from build123d import *

# Parameters (mm, degrees)
SKETCH_1_R          = 7.5
EXTRUDE_1_DEPTH     = 1
FILLET_1_R          = 3
FILLET_2_R          = 3.5
CUT_EXTRUDE_1_DEPTH = 10
EXTRUDE_2_DEPTH     = 1
FILLET_3_R          = 5


with BuildPart() as part:
    # 草图1 → 凸台-拉伸1 (new body)
    with BuildSketch(Plane.XY):
        with BuildLine():
            Line((-34, 37.637190605), (-34, 37.66227766))
            ThreePointArc((-34, 37.66227766), (-35.458039892, 36.370828693), (-36, 34.5))
            Line((-36, 34.5), (-36, -12))
            Line((-36, -12), (-41, -17))
            Line((-41, -17), (-41, -37))
            Line((-41, -37), (-36, -42))
            Line((-36, -42), (-36, -48.5))
            ThreePointArc((-36, -48.5), (-34.974873734, -50.974873734), (-32.5, -52))
            Line((-32.5, -52), (-3, -52))
            Line((-3, -52), (27, -52))
            Line((27, -52), (27, -30.660254038))
            Line((27, -30.660254038), (22, -22))
            Line((22, -22), (22, -2))
            Line((22, -2), (22, 37.977350269))
            Line((22, 37.977350269), (-32.5, 37.977350269))
            ThreePointArc((-32.5, 37.977350269), (-33.269043009, 37.891244277), (-34, 37.637190605))
        make_face()
        Circle(SKETCH_1_R, mode=Mode.SUBTRACT)
        with BuildLine():
            Line((-38, -34.5), (-37, -34.5))
            ThreePointArc((-37, -34.5), (-36.292893219, -34.207106781), (-36, -33.5))
            Line((-36, -33.5), (-36, -20.5))
            ThreePointArc((-36, -20.5), (-36.292893219, -19.792893219), (-37, -19.5))
            Line((-37, -19.5), (-38, -19.5))
            ThreePointArc((-38, -19.5), (-38.707106781, -19.792893219), (-39, -20.5))
            Line((-39, -20.5), (-39, -33.5))
            ThreePointArc((-39, -33.5), (-38.707106781, -34.207106781), (-38, -34.5))
        make_face(mode=Mode.SUBTRACT)
        with BuildLine():
            Line((-14.5, -46.5), (-9.5, -46.5))
            ThreePointArc((-9.5, -46.5), (1.813708499, -41.813708499), (6.5, -30.5))
            Line((6.5, -30.5), (6.5, -24.5))
            ThreePointArc((6.5, -24.5), (1.813708499, -13.186291501), (-9.5, -8.5))
            Line((-9.5, -8.5), (-14.5, -8.5))
            ThreePointArc((-14.5, -8.5), (-25.813708499, -13.186291501), (-30.5, -24.5))
            Line((-30.5, -24.5), (-30.5, -30.5))
            ThreePointArc((-30.5, -30.5), (-25.813708499, -41.813708499), (-14.5, -46.5))
        make_face(mode=Mode.SUBTRACT)
        with BuildLine():
            Line((11.977350269, 31), (11.977350269, 18.384776311))
            ThreePointArc((11.977350269, 18.384776311), (11.370110637, 15.331976529), (9.640838471, 12.74393784))
            Line((9.640838471, 12.74393784), (7.791596066, 10.894695435))
            ThreePointArc((7.791596066, 10.894695435), (7.199175676, 9.464466094), (7.791596066, 8.034236753))
            Line((7.791596066, 8.034236753), (8.498702848, 7.327129972))
            ThreePointArc((8.498702848, 7.327129972), (9.928932188, 6.734709582), (11.359161529, 7.327129972))
            Line((11.359161529, 7.327129972), (14.672870028, 10.640838471))
            ThreePointArc((14.672870028, 10.640838471), (16.411961883, 13.243573363), (17.022649731, 16.313708499))
            Line((17.022649731, 16.313708499), (17.022649731, 31))
            ThreePointArc((17.022649731, 31), (16.430229341, 32.430229341), (15, 33.022649731))
            Line((15, 33.022649731), (14, 33.022649731))
            ThreePointArc((14, 33.022649731), (12.569770659, 32.430229341), (11.977350269, 31))
        make_face(mode=Mode.SUBTRACT)
        with BuildLine():
            Line((7, 33.022649731), (2, 33.022649731))
            ThreePointArc((2, 33.022649731), (0.569770659, 32.430229341), (-0.022649731, 31))
            Line((-0.022649731, 31), (-0.022649731, 12.328427125))
            ThreePointArc((-0.022649731, 12.328427125), (1.225965459, 10.459742437), (3.430229341, 10.898197784))
            Line((3.430229341, 10.898197784), (6.672870028, 14.140838471))
            ThreePointArc((6.672870028, 14.140838471), (8.411961883, 16.743573363), (9.022649731, 19.813708499))
            Line((9.022649731, 19.813708499), (9.022649731, 31))
            ThreePointArc((9.022649731, 31), (8.430229341, 32.430229341), (7, 33.022649731))
        make_face(mode=Mode.SUBTRACT)
        with BuildLine():
            Line((-6.430229341, 22.359161529), (-30.430229341, -1.640838471))
            ThreePointArc((-30.430229341, -1.640838471), (-30.861813207, -2.280647977), (-31.022337577, -3.035533906))
            ThreePointArc((-31.022337577, -3.035533906), (-30.41761054, -4.442737776), (-29, -5.022649731))
            Line((-29, -5.022649731), (-22.928932188, -5.022649731))
            ThreePointArc((-22.928932188, -5.022649731), (-19.858797052, -4.411961883), (-17.25606216, -2.672870028))
            Line((-17.25606216, -2.672870028), (-5.327129972, 9.25606216))
            ThreePointArc((-5.327129972, 9.25606216), (-3.588038117, 11.858797052), (-2.977350269, 14.928932188))
            Line((-2.977350269, 14.928932188), (-2.977350269, 20.928932188))
            ThreePointArc((-2.977350269, 20.928932188), (-4.225965459, 22.797616876), (-6.430229341, 22.359161529))
        make_face(mode=Mode.SUBTRACT)
        with BuildLine():
            Line((-27.569770659, 5.398197784), (-3.569770659, 29.398197784))
            ThreePointArc((-3.569770659, 29.398197784), (-3.131315312, 30.054392583), (-2.977350269, 30.828427125))
            Line((-2.977350269, 30.828427125), (-2.977350269, 31))
            ThreePointArc((-2.977350269, 31), (-3.569770659, 32.430229341), (-5, 33.022649731))
            Line((-5, 33.022649731), (-23, 33.022649731))
            ThreePointArc((-23, 33.022649731), (-28.672870028, 30.672870028), (-31.022649731, 25))
            Line((-31.022649731, 25), (-31.022649731, 6.828427125))
            ThreePointArc((-31.022649731, 6.828427125), (-29.774034541, 4.959742437), (-27.569770659, 5.398197784))
        make_face(mode=Mode.SUBTRACT)
    extrude(amount=EXTRUDE_1_DEPTH)

    # 圆角1
    fillet_1_edges = [part.edges().sort_by_distance(p)[0] for p in [
        (22, -22, 0.5),
        (27, -30.660254038, 0.5),
    ]]
    fillet(fillet_1_edges, radius=FILLET_1_R)

    # 圆角2
    fillet_2_edges = [part.edges().sort_by_distance(p)[0] for p in [
        (22, 37.977350269, 0.5),
        (27, -52, 0.5),
    ]]
    fillet(fillet_2_edges, radius=FILLET_2_R)

    # 草图2 → 切除-拉伸1 (cut)
    with BuildSketch(Plane(origin=(0, 0, 0), x_dir=(-1, 0, 0), z_dir=(0, 0, -1))):
        with BuildLine():
            Line((-22.51, -47), (-22.49, -47))
            ThreePointArc((-22.49, -47), (-20.729304115, -46.270695885), (-20, -44.51))
            Line((-20, -44.51), (-20, -34.49))
            ThreePointArc((-20, -34.49), (-20.729304115, -32.729304115), (-22.49, -32))
            Line((-22.49, -32), (-22.51, -32))
            ThreePointArc((-22.51, -32), (-24.270695885, -32.729304115), (-25, -34.49))
            Line((-25, -34.49), (-25, -44.51))
            ThreePointArc((-25, -44.51), (-24.270695885, -46.270695885), (-22.51, -47))
        make_face()
    extrude(amount=-CUT_EXTRUDE_1_DEPTH, mode=Mode.SUBTRACT)

    # 草图3 → 凸台-拉伸2 (add)
    with BuildSketch(Plane(origin=(0, 0, 0), x_dir=(-1, 0, 0), z_dir=(0, 0, -1))):
        with BuildLine():
            Line((12, -27.5), (29.320508076, -17.5))
            ThreePointArc((29.320508076, -17.5), (30.076804592, -18.942597605), (30.713203436, -20.441953728))
            Line((30.713203436, -20.441953728), (30.713203436, -10.922424267))
            Line((30.713203436, -10.922424267), (2, -27.5))
            Line((2, -27.5), (30.713203436, -44.077575733))
            Line((30.713203436, -44.077575733), (30.713203436, -34.558046272))
            ThreePointArc((30.713203436, -34.558046272), (30.076804592, -36.057402395), (29.320508076, -37.5))
            Line((29.320508076, -37.5), (12, -27.5))
        make_face()
    extrude(amount=-EXTRUDE_2_DEPTH)

    # 圆角3
    fillet_3_edges = [part.edges().sort_by_distance(p)[0] for p in [
        (-26.164686329, -41.451488157, 0.5),
        (-28.98117459, -37.304085721, 0.5),
        (-28.98117459, -17.695914279, 0.5),
        (-26.164686329, -13.548511843, 0.5),
        (-12, -27.5, 0.5),
        (-2, -27.5, 0.5),
    ]]
    fillet(fillet_3_edges, radius=FILLET_3_R)


solid = part.part
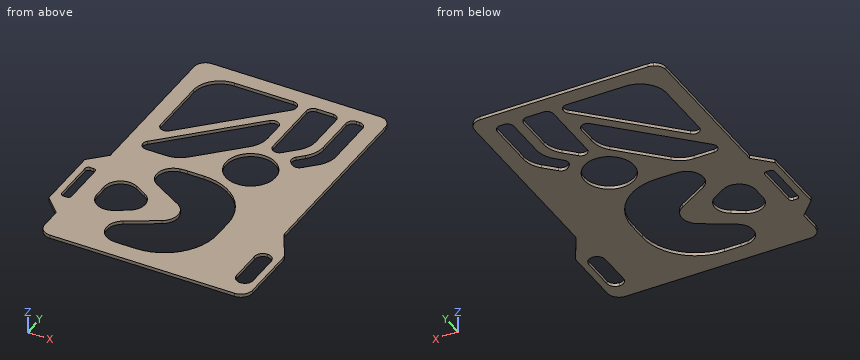
Design review of the part built by this model. Coordinates are the model's own, in mm. Round coordinates to 2 decimals unless told otherwise and drop trailing zeros. Loops run counter-clockwise (first coordinate to the right, second up) from the corner with the lowest first, then second, coordinate; pieces in that order, holes last. Notation, with made-up numbers: (25, 87.5) -> (49, 87.5) arc R21 ccw to (49, 101.5) -> close; hole circle Ø9 at (50, 64.25). An arc over 180 degrees is marked (long way). Use one line per item in the form item = value. Start each with the question number.
Q1. We need section D-D on y = 32. Give the boundary of the cut face in (x, z).
Q2. Wall thickness on line 1 along Y through (x, z) = (-27, 0.75); line 2 along X through (y, z) = (27, 0.5); line 3 along X through (y, z) = (8.5, 0.9): over which ranges is each line inside the solid? List them lowest first. Write a range as [from, to].
Q3. We need section A-A on y = 0. Give the boundary of the cut face in (x, z), then the cut area to 3 significant figures.
Q4. We need section B-B on x = -13.5. Give the boundary of the cut face in (y, z), then the cut area to 3 significant figures.
Q5. We need section C-C on x = 21. Give the boundary of the cut face in (y, z) (3 decimals).
Calculated:
q1.outline = (-36, 0) -> (-26.92, 0) -> (-26.92, 1) -> (-36, 1) -> close; (-3.24, 0) -> (0.24, 0) -> (0.24, 1) -> (-3.24, 1) -> close; (8.76, 0) -> (12.24, 0) -> (12.24, 1) -> (8.76, 1) -> close; (16.76, 0) -> (22, 0) -> (22, 1) -> (16.76, 1) -> close
q2.line_1 = [-52, -34.29], [-20.71, -5.02], [1.79, 5.97], [31.95, 37.98]
q2.line_2 = [-36, -30.77], [-5.97, -0.02], [9.02, 11.98], [17.02, 22]
q2.line_3 = [-36, -31.02], [-24.47, -20.29], [-6.08, 7.44], [12.53, 22]
q3.outline = (-36, 0) -> (-28.79, 0) -> (-28.79, 1) -> (-36, 1) -> close; (-14.58, 0) -> (-7.5, 0) -> (-7.5, 1) -> (-14.58, 1) -> close; (7.5, 0) -> (22, 0) -> (22, 1) -> (7.5, 1) -> close
q3.area = 28.8 mm²
q4.outline = (-52, 0) -> (-46.5, 0) -> (-46.5, 1) -> (-52, 1) -> close; (-34.14, 0) -> (-20.86, 0) -> (-20.86, 1) -> (-34.14, 1) -> close; (-8.5, 0) -> (1.08, 0) -> (1.08, 1) -> (-8.5, 1) -> close; (15.29, 0) -> (19.47, 0) -> (19.47, 1) -> (15.29, 1) -> close; (33.02, 0) -> (37.98, 0) -> (37.98, 1) -> (33.02, 1) -> close
q4.area = 37.5 mm²
q5.outline = (-52, 0) -> (-46.505, 0) -> (-46.505, 1) -> (-52, 1) -> close; (-32.495, 0) -> (36.927, 0) -> (36.927, 1) -> (-32.495, 1) -> close
